from build123d import *

# Parameters (mm, degrees)
SKETCH_1_R      = 56
SKETCH_1_R_2    = 2.15
SKETCH_1_R_3    = 44.5
EXTRUDE_1_DEPTH = 6


with BuildPart() as part:
    # 草图1 → 凸台-拉伸1 (new body)
    with BuildSketch(Plane(origin=(0, 0, 0), x_dir=(-1, 0, 0), z_dir=(0, 0, -1))):
        with Locations(Location((0, 0, 0), (0, 0, 180))):
            Circle(SKETCH_1_R)
        with Locations(Location((11.126046698, 48.746395609, 0), (0, 0, 180))):
            Circle(SKETCH_1_R_2, mode=Mode.SUBTRACT)
        with Locations(Location((21.694186956, 45.048443395, 0), (0, 0, 180))):
            Circle(SKETCH_1_R_2, mode=Mode.SUBTRACT)
        with Locations(Location((31.174490093, 39.091574123, 0), (0, 0, 180))):
            Circle(SKETCH_1_R_2, mode=Mode.SUBTRACT)
        with Locations(Location((39.091574123, 31.174490093, 0), (0, 0, 180))):
            Circle(SKETCH_1_R_2, mode=Mode.SUBTRACT)
        with Locations(Location((45.048443395, 21.694186956, 0), (0, 0, 180))):
            Circle(SKETCH_1_R_2, mode=Mode.SUBTRACT)
        with Locations(Location((48.746395609, 11.126046698, 0), (0, 0, 180))):
            Circle(SKETCH_1_R_2, mode=Mode.SUBTRACT)
        with Locations(Location((50, 0, 0), (0, 0, 180))):
            Circle(SKETCH_1_R_2, mode=Mode.SUBTRACT)
        with Locations(Location((48.746395609, -11.126046698, 0), (0, 0, 180))):
            Circle(SKETCH_1_R_2, mode=Mode.SUBTRACT)
        with Locations(Location((45.048443395, -21.694186956, 0), (0, 0, 180))):
            Circle(SKETCH_1_R_2, mode=Mode.SUBTRACT)
        with Locations(Location((39.091574123, -31.174490093, 0), (0, 0, 180))):
            Circle(SKETCH_1_R_2, mode=Mode.SUBTRACT)
        with Locations(Location((31.174490093, -39.091574123, 0), (0, 0, 180))):
            Circle(SKETCH_1_R_2, mode=Mode.SUBTRACT)
        with Locations(Location((21.694186956, -45.048443395, 0), (0, 0, 180))):
            Circle(SKETCH_1_R_2, mode=Mode.SUBTRACT)
        with Locations(Location((11.126046698, -48.746395609, 0), (0, 0, 180))):
            Circle(SKETCH_1_R_2, mode=Mode.SUBTRACT)
        with Locations(Location((0, -50, 0), (0, 0, 180))):
            Circle(SKETCH_1_R_2, mode=Mode.SUBTRACT)
        with Locations(Location((-11.126046698, -48.746395609, 0), (0, 0, 180))):
            Circle(SKETCH_1_R_2, mode=Mode.SUBTRACT)
        with Locations(Location((-21.694186956, -45.048443395, 0), (0, 0, 180))):
            Circle(SKETCH_1_R_2, mode=Mode.SUBTRACT)
        with Locations(Location((-31.174490093, -39.091574123, 0), (0, 0, 180))):
            Circle(SKETCH_1_R_2, mode=Mode.SUBTRACT)
        with Locations(Location((-39.091574123, -31.174490093, 0), (0, 0, 180))):
            Circle(SKETCH_1_R_2, mode=Mode.SUBTRACT)
        with Locations(Location((-45.048443395, -21.694186956, 0), (0, 0, 180))):
            Circle(SKETCH_1_R_2, mode=Mode.SUBTRACT)
        with Locations(Location((-48.746395609, -11.126046698, 0), (0, 0, 180))):
            Circle(SKETCH_1_R_2, mode=Mode.SUBTRACT)
        with Locations(Location((-50, 0, 0), (0, 0, 180))):
            Circle(SKETCH_1_R_2, mode=Mode.SUBTRACT)
        with Locations(Location((-48.746395609, 11.126046698, 0), (0, 0, 180))):
            Circle(SKETCH_1_R_2, mode=Mode.SUBTRACT)
        with Locations(Location((-45.048443395, 21.694186956, 0), (0, 0, 180))):
            Circle(SKETCH_1_R_2, mode=Mode.SUBTRACT)
        with Locations(Location((-39.091574123, 31.174490093, 0), (0, 0, 180))):
            Circle(SKETCH_1_R_2, mode=Mode.SUBTRACT)
        with Locations(Location((-31.174490093, 39.091574123, 0), (0, 0, 180))):
            Circle(SKETCH_1_R_2, mode=Mode.SUBTRACT)
        with Locations(Location((-21.694186956, 45.048443395, 0), (0, 0, 180))):
            Circle(SKETCH_1_R_2, mode=Mode.SUBTRACT)
        with Locations(Location((-11.126046698, 48.746395609, 0), (0, 0, 180))):
            Circle(SKETCH_1_R_2, mode=Mode.SUBTRACT)
        with Locations(Location((0, 50, 0), (0, 0, 180))):
            Circle(SKETCH_1_R_2, mode=Mode.SUBTRACT)
        with Locations(Location((0, 0, 0), (0, 0, 180))):
            Circle(SKETCH_1_R_3, mode=Mode.SUBTRACT)
    extrude(amount=-EXTRUDE_1_DEPTH)


solid = part.part
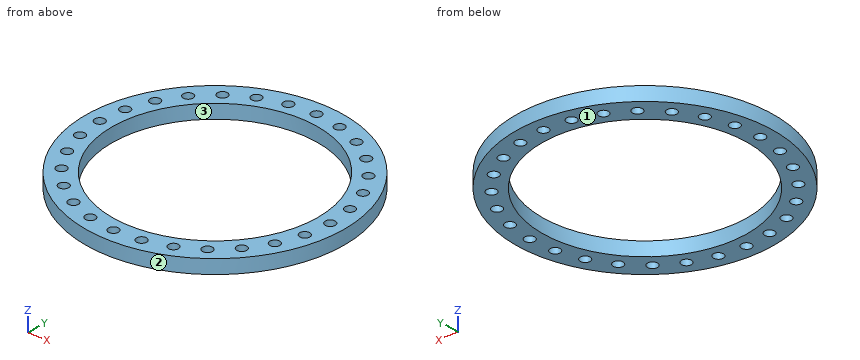
Read the model definition and answer for the solid it produces. Units are mm, in the model's axes. Face numbers are marked on the shaded views. Give positions to 0.01 mm unless a question says otherwise; leave off trailing zeros. Write each loop counter-clockwise with the first axis right and the second up, starting at its lowest first coordinate (ties: lowest second). Pieces come first, ordered by that corner, then holes. Notation, with made-up numbers: (43.25, 43.25) -> (62.25, 43.25) arc R19 ccw to (62.25, 71.25) -> close; hole circle Ø6 at (86, -39.75). An arc over 180 degrees is marked (long way). Answer as a JSON object with one key per item and string values. Group by question number.
1) Consider L1, parallel to Y at x = 0, z = 3.35; L2, parallel to Y at x = 11, z = 4.2; L3, parallel to Y at x = 47.5, z = 5.4. Determine where each line is inside the solid, lowest interval first. Write a range as from..to.
2) Each of these flat-tipped pins is pushed along its axis until it touches: P1, Ø7, axis at x = -50, y = 0, coming from the +Z side; P2, Ø2, axis at x = -22.5, z = 1.5, coming from the -Y side; P3, Ø3, axis at y = -37, z = 1.5, coming from the +X side; P4, Ø1, axis at x = 4, z = 1, coming from the +Y side. Where does it stop, or does it pass through?
3) Find section A-A (y = 0). Write down the section's boundary in (x, z).
4) Find section C-C (x = 16.5). Write down the section's boundary in (y, z), and give its area (3 significant figures).
5) The mould has two halves that part along Y. Classify the marked faces 1, 2 and 3: +Y half, -Y half, draft (parallel to the pull), parting line (faces both ways), or undercut.
6) Find section B-B (x = 31). Write down the section's boundary in (y, z), and give its area (3 significant figures).
7) Find section D-D (z = 4.9). Count the separate pieces of the cut face and the enclosed holes in it, and give its area (3 significant figures).
Values follow:
{
 "1": {"L1": "y = -56..-52.15, -47.85..-44.5, 44.5..47.85, 52.15..56", "L2": "y = -54.91..-50.89, -46.6..-43.12, 43.12..46.6, 50.89..54.91", "L3": "y = -29.66..-12.88, -9.37..9.37, 12.88..29.66"},
 "2": {"P1": "stops at z = 6", "P2": "stops at y = -51.71", "P3": "stops at x = 43.31", "P4": "stops at y = 55.89"},
 "3": {"outline": "(-56, 0) -> (-52.15, 0) -> (-52.15, 6) -> (-56, 6) -> close; (-47.85, 0) -> (-44.5, 0) -> (-44.5, 6) -> (-47.85, 6) -> close; (44.5, 0) -> (47.85, 0) -> (47.85, 6) -> (44.5, 6) -> close; (52.15, 0) -> (56, 0) -> (56, 6) -> (52.15, 6) -> close"},
 "4": {"outline": "(-53.51, 0) -> (-41.33, 0) -> (-41.33, 6) -> (-53.51, 6) -> close; (41.33, 0) -> (53.51, 0) -> (53.51, 6) -> (41.33, 6) -> close", "area": "146 mm2"},
 "5": {"face 1": "draft", "face 2": "parting line", "face 3": "undercut"},
 "6": {"outline": "(-46.64, 0) -> (-41.23, 0) -> (-41.23, 6) -> (-46.64, 6) -> close; (-36.95, 0) -> (-31.93, 0) -> (-31.93, 6) -> (-36.95, 6) -> close; (31.93, 0) -> (36.95, 0) -> (36.95, 6) -> (31.93, 6) -> close; (41.23, 0) -> (46.64, 0) -> (46.64, 6) -> (41.23, 6) -> close", "area": "125 mm2"},
 "7": {"separate pieces": "1", "enclosed holes": "29", "area": "3,220 mm2"}
}
